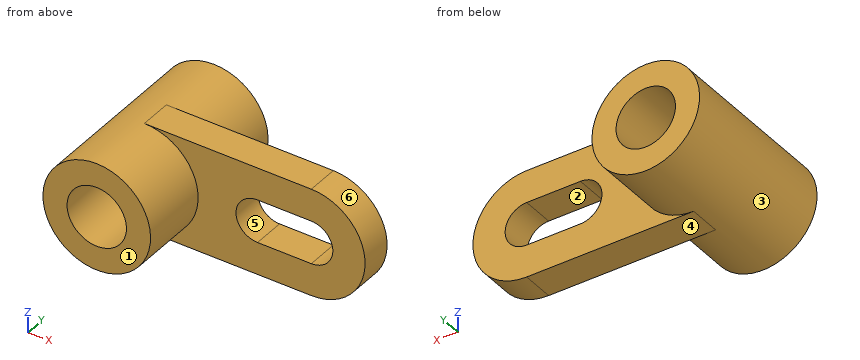
from build123d import *

# Parameters (mm, degrees)
BOSS_EXTRUDE1_DEPTH      = 19.05
CUT_EXTRUDE3_DEPTH       = 20.05
SKETCH3_R                = 31.75
BOSS_EXTRUDE2_DEPTH      = 41.402
BOSS_EXTRUDE2_DEPTH_BACK = 60.198
SKETCH4_R                = 17.526
CUT_EXTRUDE2_DEPTH       = 102.6


with BuildPart() as part:
    # Sketch1 → Boss-Extrude1 (new body)
    with BuildSketch(Plane(origin=(0, 0, 0), x_dir=(1, 0, 0), z_dir=(0, 1, 0))):
        with BuildLine():
            Line((-49.276, 31.75), (49.276, 31.75))
            ThreePointArc((49.276, 31.75), (81.026, 0), (49.276, -31.75))
            Line((49.276, -31.75), (-49.276, -31.75))
            ThreePointArc((-49.276, -31.75), (-81.026, 0), (-49.276, 31.75))
        make_face()
    extrude(amount=BOSS_EXTRUDE1_DEPTH)

    # Sketch5 → Cut-Extrude3 (cut, through all)
    with BuildSketch(Plane.XZ):
        with BuildLine():
            Line((17.526, 12.7), (49.276, 12.7))
            ThreePointArc((49.276, 12.7), (61.976, 0), (49.276, -12.7))
            Line((49.276, -12.7), (17.526, -12.7))
            ThreePointArc((17.526, -12.7), (4.826, 0), (17.526, 12.7))
        make_face()
    extrude(amount=-CUT_EXTRUDE3_DEPTH, mode=Mode.SUBTRACT)

    # Sketch3 → Boss-Extrude2 (add, two sides)
    with BuildSketch(Plane(origin=(0, 19.05, 0), x_dir=(1, 0, 0), z_dir=(0, 1, 0))) as boss_extrude2_sk:
        with Locations(Location((-49.276, 0, 0), (0, 0, 270))):  # turned: the seam where the file's is
            Circle(SKETCH3_R)
    extrude(amount=BOSS_EXTRUDE2_DEPTH)
    extrude(boss_extrude2_sk.sketch, amount=-BOSS_EXTRUDE2_DEPTH_BACK)

    # Sketch4 → Cut-Extrude2 (cut, through all)
    with BuildSketch(Plane(origin=(0, 60.452, 0), x_dir=(1, 0, 0), z_dir=(0, 1, 0))):
        with Locations(Location((-49.276, 0, 0), (0, 0, 270))):  # turned: the seam where the file's is
            Circle(SKETCH4_R)
    extrude(amount=-CUT_EXTRUDE2_DEPTH, mode=Mode.SUBTRACT)


solid = part.part
Model file for the job. Use its own axes, mm. Face numbers are marked on the shaded views. A direction names the side the tool comes from. Give positions to 0.01 mm unless a question says otherwise; leave off trailing zeros. Loops run counter-clockwise (first coordinate to the right, second up) from the corner with the lowest first, then second, coordinate; pieces in that order, holes last.
Item 1: Slice it at A-A (z = 0). Write the cut outline in (x, y), plus the area to 3 significant figures.
Check values:
outline: (-81.03, -41.15) - (-66.8, -41.15) - (-66.8, 60.45) - (-81.03, 60.45) - close; (-31.75, -41.15) - (-17.53, -41.15) - (-17.53, 0) - (4.83, 0) - (4.83, 19.05) - (-17.53, 19.05) - (-17.53, 60.45) - (-31.75, 60.45) - close; (61.98, 0) - (81.03, 0) - (81.03, 19.05) - (61.98, 19.05) - close
area: 3,680 mm2
Item 2: Mould opens along Z. For the marked faces 4, 5 and 6 say: +Z half, -Z half, draft (parallel to the pull), parting line (faces both ways), or undercut.
Check values:
face 4: -Z half
face 5: undercut
face 6: parting line
Item 3: Slice it at C-C (y = 34.5). Write the cut outline in (x, z).
Check values:
outline: circle Ø63.5 at (-49.28, 0); hole circle Ø35.05 at (-49.28, 0)
Item 4: Drill centre lines: line 1 along X through (y, z) = (23.5, 0); line 2 along X through (y, z) = (16.5, 0); line 3 along Z through (x, y) = (26, 3). Where is each one in solid material? Low to high.
Check values:
line 1: x = -81.03 to -66.8, -31.75 to -17.53
line 2: x = -81.03 to -66.8, -31.75 to 4.83, 61.98 to 81.03
line 3: z = -31.75 to -12.7, 12.7 to 31.75
Item 5: Drop flat-ended pins along their axis: P1, Ø2, axis at x = -23.5, z = 22.5, coming from the -Y side; P2, Ø10, axis at x = -57.5, y = 6.5, coming from the +Z side; P3, Ø5, axis at x = -34.5, y = -29, coming from the -Z side. Give the stop position or say it passes through.
Check values:
P1: stops at y = 0
P2: stops at z = 31.59
P3: stops at z = -29.28
Item 6: Slice it at B-B (x = 45). Write the cut outline in (y, z).
Check values:
outline: (0, -31.75) - (19.05, -31.75) - (19.05, -12.7) - (0, -12.7) - close; (0, 12.7) - (19.05, 12.7) - (19.05, 31.75) - (0, 31.75) - close
Item 7: Which spindle directions (+Z, -Z, +X, -X, +Y, -Y) get a long thin tool onto all of the face, cutting with end or side? Do the marked faces 1, 2 and 3. Say none if no direction does.
Check values:
face 1: +Z, -Z, +X, -X, -Y
face 2: +Y, -Y
face 3: none
Item 8: Slice it at D-D (z = 26.5). Write the cut outline in (x, y), plus the area to 3 significant figures.
Check values:
outline: (-66.76, -41.15) - (-31.79, -41.15) - (-31.79, 0) - (66.76, 0) - (66.76, 19.05) - (-31.79, 19.05) - (-31.79, 60.45) - (-66.76, 60.45) - close
area: 5,430 mm2
